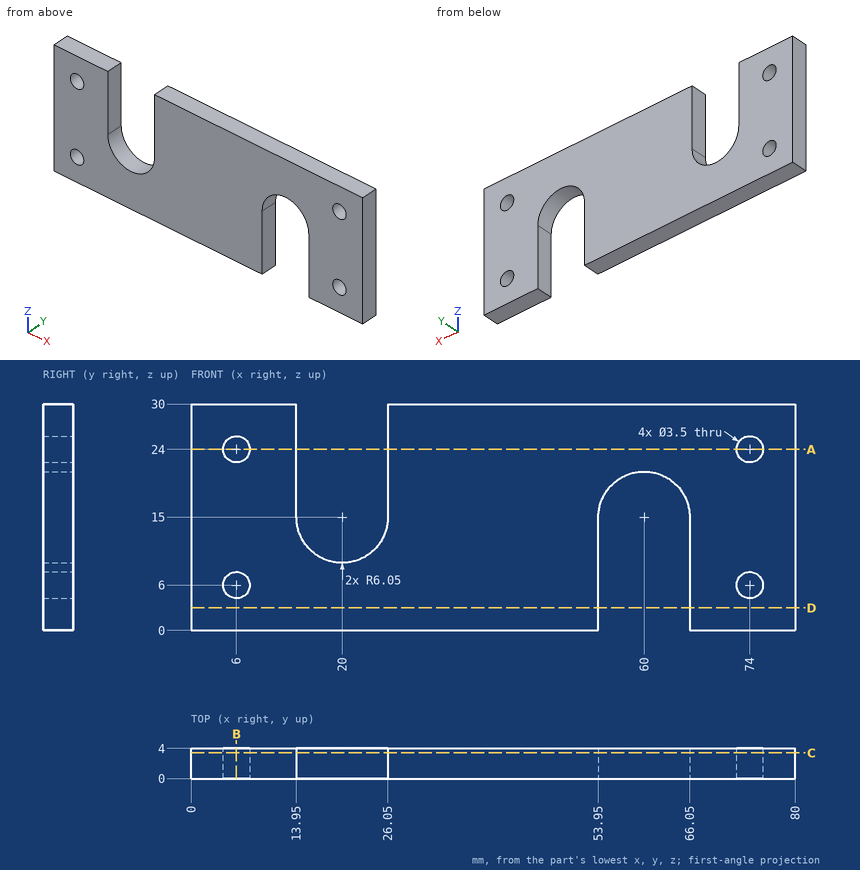
Study the drawing (mm; zero at the part's minimum x, y, z) and answer. Give positions to 0.01 mm unless a question says otherwise; leave off trailing zeros. Loops run counter-clockwise (first coordinate to the right, second up) from the corner with the lowest first, then second, coordinate; pieces in that order, holes last. Notation, with made-up numbers: (18.5, -38.5) -> (24.5, -38.5) arc R5 cw to (24.5, -29.5) -> close; hole circle Ø1 at (-38.5, 29). An arc over 180 degrees is marked (long way). Write item = value, one per line. Start each with the question number.
(1) Find section A-A on z = 24. Give the vertices of the cut face in (x, y), and give its area (3 significant figures).
(2) Find the intervals of material crossed by probe 1 along X at (y, z) = (2.2, 6); probe 2 along Z at (x, y) = (74, 2.25); probe 3 along X at (y, z) = (1.5, 24), in increasing order. Write a range as from..to.
(3) Find section B-B on x = 6. Give the vertices of the cut face in (y, z).
(4) Find section D-D on z = 3. Give the vertices of the cut face in (x, y).
(5) Find section C-C on y = 3.4. Give the vertices of the cut face in (x, z).
From the geometry:
q1.outline = (0, 0) -> (4.25, 0) -> (4.25, 4) -> (0, 4) -> close; (7.75, 0) -> (13.95, 0) -> (13.95, 4) -> (7.75, 4) -> close; (26.05, 0) -> (72.25, 0) -> (72.25, 4) -> (26.05, 4) -> close; (75.75, 0) -> (80, 0) -> (80, 4) -> (75.75, 4) -> close
q1.area = 244 mm^2
q2.probe_1 = 0..4.25, 7.75..53.95, 66.05..72.25, 75.75..80
q2.probe_2 = 0..4.25, 7.75..22.25, 25.75..30
q2.probe_3 = 0..4.25, 7.75..13.95, 26.05..72.25, 75.75..80
q3.outline = (0, 0) -> (4, 0) -> (4, 4.25) -> (0, 4.25) -> close; (0, 7.75) -> (4, 7.75) -> (4, 22.25) -> (0, 22.25) -> close; (0, 25.75) -> (4, 25.75) -> (4, 30) -> (0, 30) -> close
q4.outline = (0, 0) -> (53.95, 0) -> (53.95, 4) -> (0, 4) -> close; (66.05, 0) -> (80, 0) -> (80, 4) -> (66.05, 4) -> close
q5.outline = (0, 0) -> (53.95, 0) -> (53.95, 15) arc R6.05 cw to (66.05, 15) -> (66.05, 0) -> (80, 0) -> (80, 30) -> (26.05, 30) -> (26.05, 15) arc R6.05 cw to (13.95, 15) -> (13.95, 30) -> (0, 30) -> close; hole circle Ø3.5 at (6, 6); hole circle Ø3.5 at (6, 24); hole circle Ø3.5 at (74, 6); hole circle Ø3.5 at (74, 24)
